from build123d import *

# Parameters (mm, degrees)
F0_W      = 539.75
F0_H      = 552.45
F1_DEPTH  = 3.175
F3_DEPTH  = 58.7375
F4_W      = 539.75
F4_H      = 127
F4_R      = 4.7625
F5_DEPTH  = 3.175
F6_R      = 4.699
F7_DEPTH  = 17.145
F8_R      = 25.4
F9_DEPTH  = 1.651
F10_W     = 76.2
F10_H     = 31.75
F11_DEPTH = 107.8865
F12_R     = 38.09999
F13_W     = 3.175
F13_H     = 546.1
F14_DEPTH = 31.75


# Not quite as in the source:
# - a fillet or chamfer is up to 0.001 mm smaller than in the source, because OpenCascade refuses the exact size


with BuildPart() as f1:
    # F0 (on Top) → F1 (new body)
    with BuildSketch(Plane.XY):
        Rectangle(F0_W, F0_H)
        with BuildLine():
            ThreePointArc((-219.075, -98.425), (-217.2151280605, -93.9348719395), (-212.725, -92.075))
            Line((-212.725, -92.075), (-203.2, -92.075))
            ThreePointArc((-203.2, -92.075), (-198.7098719395, -93.9348719395), (-196.85, -98.425))
            Line((-196.85, -98.425), (-196.85, -193.675))
            ThreePointArc((-196.85, -193.675), (-198.7098719395, -198.1651280605), (-203.2, -200.025))
            Line((-203.2, -200.025), (-212.725, -200.025))
            ThreePointArc((-212.725, -200.025), (-217.2151280605, -198.1651280605), (-219.075, -193.675))
            Line((-219.075, -193.675), (-219.075, -98.425))
        make_face(mode=Mode.SUBTRACT)
        with BuildLine():
            ThreePointArc((-219.075, 193.675), (-217.2151280605, 198.1651280605), (-212.725, 200.025))
            Line((-212.725, 200.025), (-206.375, 200.025))
            ThreePointArc((-206.375, 200.025), (-201.8848719395, 198.1651280605), (-200.025, 193.675))
            Line((-200.025, 193.675), (-200.025, 104.775))
            ThreePointArc((-200.025, 104.775), (-201.8848719395, 100.2848719395), (-206.375, 98.425))
            Line((-206.375, 98.425), (-212.725, 98.425))
            ThreePointArc((-212.725, 98.425), (-217.2151280605, 100.2848719395), (-219.075, 104.775))
            Line((-219.075, 104.775), (-219.075, 193.675))
        make_face(mode=Mode.SUBTRACT)
    extrude(amount=F1_DEPTH)

    # F2 (on face) → F3 (join)
    with BuildSketch(Plane.XY.offset(3.175)):
        Polygon((-269.875, 276.225), (-269.875, 273.05), (266.7, 273.05), (266.7, -273.05), (-269.875, -273.05), (-269.875, -276.225), (269.875, -276.225), (269.875, 276.225), align=None)
    extrude(amount=F3_DEPTH)

    # F4 (on face) → F5 (join)
    with BuildSketch(Plane.XY.offset(61.9125)):
        with Locations((0, 336.55)):
            Rectangle(F4_W, F4_H)
        with Locations((-219.075, 349.25)):
            Circle(F4_R, mode=Mode.SUBTRACT)
        with Locations((219.075, 349.25)):
            Circle(F4_R, mode=Mode.SUBTRACT)
        with Locations((0, -336.55)):
            Rectangle(F4_W, F4_H)
        with Locations((-219.075, -349.25)):
            Circle(F4_R, mode=Mode.SUBTRACT)
        with Locations((219.075, -349.25)):
            Circle(F4_R, mode=Mode.SUBTRACT)
    extrude(amount=-F5_DEPTH)



with BuildPart() as f7:
    # F6 (on face) → F7 (new body)
    with BuildSketch(Plane(origin=(0, 0, 58.7375), x_dir=(1, 0, 0), z_dir=(0, 0, -1))):
        with Locations((-219.075, 349.25)):
            Circle(F6_R)
    extrude(amount=-F7_DEPTH)


with BuildPart() as f7b:
    # F6 (on face) → F7, piece 2 (new body)
    with BuildSketch(Plane(origin=(0, 0, 58.7375), x_dir=(1, 0, 0), z_dir=(0, 0, -1))):
        with Locations((219.075, 349.25)):
            Circle(F6_R)
    extrude(amount=-F7_DEPTH)


with BuildPart() as f7c:
    # F6 (on face) → F7, piece 3 (new body)
    with BuildSketch(Plane(origin=(0, 0, 58.7375), x_dir=(1, 0, 0), z_dir=(0, 0, -1))):
        with Locations((-219.075, -349.25)):
            Circle(F6_R)
    extrude(amount=-F7_DEPTH)


with BuildPart() as f7d:
    # F6 (on face) → F7, piece 4 (new body)
    with BuildSketch(Plane(origin=(0, 0, 58.7375), x_dir=(1, 0, 0), z_dir=(0, 0, -1))):
        with Locations((219.075, -349.25)):
            Circle(F6_R)
    extrude(amount=-F7_DEPTH)


with BuildPart() as f1_1:
    add(f1.part)

    add(f7.part)  # F9 merges F7

    add(f7b.part)  # F9 merges F7b

    add(f7c.part)  # F9 merges F7c

    add(f7d.part)  # F9 merges F7d
    # F8 (on face) → F9 (join)
    with BuildSketch(Plane(origin=(0, 0, 58.7375), x_dir=(1, 0, 0), z_dir=(0, 0, -1))):
        with Locations((-219.075, 349.25)):
            Circle(F8_R)
        with Locations((219.075, 349.25)):
            Circle(F8_R)
        with Locations((-219.075, -349.25)):
            Circle(F8_R)
        with Locations((219.075, -349.25)):
            Circle(F8_R)
    extrude(amount=F9_DEPTH)

    # F10 (on face) → F11 (join)
    with BuildSketch(Plane(origin=(0, 0, 57.0865), x_dir=(1, 0, 0), z_dir=(0, 0, -1))):
        with Locations((-206.375, 349.25)):
            Rectangle(F10_W, F10_H)
        with Locations((206.375, 349.25)):
            Rectangle(F10_W, F10_H)
        with Locations((-206.375, -349.25)):
            Rectangle(F10_W, F10_H)
        with Locations((206.375, -349.25)):
            Rectangle(F10_W, F10_H)
    extrude(amount=F11_DEPTH)

    # F12 (radius 38.1 in the source; OpenCascade refuses exactly that, so slightly less here)
    f12_edges = [f1_1.edges().sort_by_distance(p)[0] for p in [
        (-168.275, -349.25, -50.8),
        (-244.475, -349.25, -50.8),
        (168.275, -349.25, -50.8),
        (244.475, -349.25, -50.8),
        (-244.475, 349.25, -50.8),
        (-168.275, 349.25, -50.8),
        (168.275, 349.25, -50.8),
        (244.475, 349.25, -50.8),
    ]]
    fillet(f12_edges, radius=F12_R)

    # F13 (on face) → F14 (join)
    with BuildSketch(Plane.XY.offset(3.175)):
        with Locations((-268.2875, 0)):
            Rectangle(F13_W, F13_H)
    extrude(amount=-F14_DEPTH)


solid = f1_1.part
Part model, mm, in its own coordinate system. A direction names the side the tool comes from. Give positions to 0.01 mm unless a question says otherwise; leave off trailing zeros. Order: outer loops, then holes, each group sorted by start corner. A loop starts at its lowest first (then second) coordinate and runs counter-clockwise, first axis right, second up. Notation, with made-up numbers: (79.5, -18.75) -> (136.5, -18.75) arc R10 cw to (136.5, 0.25) -> close; hole circle Ø1 at (-15, 80.5). An arc over 180 degrees is marked (long way). Use one line per item in the form item = value.
(1) Pull direction X, two halves, no side cores. Call faces 5 (the face through (-266.7, -4, -14)), 6 (the face through (168.275, -349, 23)), 7 (the face through (266.7, 4, 32)): +X half, -X half, draft (parallel to the pull), parting line (faces both ways), or undercut.
Solution:
face_5 = +X half
face_6 = undercut
face_7 = -X half
(2) Drill centre lines: line 1 (Y direction, x = -238, z = 17.5) (3 decimals); line 2 (Y direction, x = -96.5, z = 53) (3 decimals); line 3 (Y direction, x = -232, z = -14.5) (3 decimals). Where is each one in solid material? Low to high. Write a range as from..to.
Solution:
line_1 = -365.125..-333.375, -276.225..-273.05, 273.05..276.225, 333.375..365.125
line_2 = -276.225..-273.05, 273.05..276.225
line_3 = -365.125..-333.375, 333.375..365.125
(3) Flat gauge pins, fed straight in: P1, Ø10, axis at y = -75, z = -23.5, coming from the +X side; P2, Ø2.5, axis at x = -209.5, z = 2, coming from the -Y side (3 decimals); P3, Ø9.5, axis at y = 344.5, z = 34, coming from the +X side (3 decimals). Where does each tip first touch, or does it go through?
Solution:
P1 = -266.7
P2 = -365.125
P3 = 244.475
(4) Tool access for faces 1 (the face through (213.569, 374.046, 57.924)), 2 (the face through (-207, -333.375, 4)), 3 (the face through (179.1, -349.5, -39.3)), 4 (the face through (2, -273.05, 32)): list every direction of +Z, -Z, +X, -X, +Y, -Y with a clear straight run to the whole face (end or side of a thin tool).
Solution:
face_1 = none
face_2 = -Z, +X, -X
face_3 = -Z, +Y, -Y
face_4 = +Z, -X
(5) Saw through at C-C (y = 115). Write the cut outline in (x, z) (1 decimal), then the cut area to 3 significant figures.
Solution:
outline = (-269.9, -28.6) -> (-266.7, -28.6) -> (-266.7, 0) -> (-219.1, 0) -> (-219.1, 3.2) -> (-269.9, 3.2) -> close; (-200, 0) -> (269.9, 0) -> (269.9, 61.9) -> (266.7, 61.9) -> (266.7, 3.2) -> (-200, 3.2) -> close
area = 1,930 mm²
